CAD build for the part. Positions are in the model's coordinates, mm. A direction names the side the tool comes from. Coordinates: 2 decimals unless noted, no trailing zeros. Loops run counter-clockwise (first coordinate to the right, second up) from the corner with the lowest first, then second, coordinate; pieces in that order, holes last.
1) Which spindle directions (+Z, -Z, +X, -X, +Y, -Y) get a long thin tool onto all of the face, cutting with end or side? Do faces 1 (the flat face through (-14, 49.431, 5)), 2 (the flat face through (-1, -10, 10)), 3 (the flat face through (39, 49.431, 5)), 4 (the flat face through (-38, 49.431, 5)). Say none if no direction does.
2) Saw through at C-C, the plane x = -42. Write the cut outline in (y, z), and give its area (3 significant figures).
3) Two-plate mould, pull along Y, no slides. Class faces 5 (the flat face through (0, 8, 12)), 6 (the cylindrical face through (8.41, 44.34, 10.99)), 7 (the flat face through (-1, -49.431, 5)): +Y half, -Y half, draft (parallel to the pull), parting line (faces both ways), or undercut.
4) Saw through at A-A, the plane z = 3.25. Write the cut outline in (x, y), and give its area (3 significant figures).
5) Wall check: line 1 along X through (y, z) = (3, 10.5); line 2 along X through (y, z) = (4.5, 10.25); line 3 along Y through (x, z) = (13, 6.75). Give the ranges that are in metal, low to high.
6) Saw through at B-B, the plane y = 2. Write the cut outline in (x, z).
7) Saw through at D-D, the plane y = -42. Write the cut outline in (x, z).
8) Pin check, flat tips, straight feed: pin 1 Ø4 at (y, z) = (61.5, 8.5) entering from -X; pin 2 Ø6.5 at (x, z) = (14.5, 5) entering from +Y; pin 3 Ø4.5 at (x, z) = (-13, 6.5) entering from +Y. Stop position of each tip, or through.
```python
from build123d import *

# Parameters (mm, degrees)
F0_W     = 103.961334
F0_H     = 98.86241
F1_DEPTH = 10
F3_DEPTH = 2
F5_DEPTH = 2
F7_DEPTH = 12


with BuildPart() as f1:
    # F0 (on Top) → F1 (new body)
    with BuildSketch(Plane.XY):
        Rectangle(F0_W, F0_H)
    extrude(amount=F1_DEPTH)

    # F2 (on face) → F3 (join)
    with BuildSketch(Plane.XY.offset(10)):
        with BuildLine():
            ThreePointArc((-16.892111, 15.737094), (-21.169771, -9.210881), (0, -23.086783))
            ThreePointArc((0, -23.086783), (21.247464, -9.030216), (16.621562, 16.022585))
            Line((16.621562, 16.022585), (14.340605, 13.488688))
            ThreePointArc((14.340605, 13.488688), (18.071472, -7.811502), (0, -19.6875))
            ThreePointArc((0, -19.6875), (-18.227079, -7.441185), (-13.778395, 14.062485))
            Line((-13.778395, 14.062485), (-16.892111, 15.737094))
        make_face()
    extrude(amount=F3_DEPTH)

    # F4 (on face) → F5 (join)
    with BuildSketch(Plane.XY.offset(10)):
        with BuildLine():
            ThreePointArc((-3.965827, -3.950249), (-3.095911, -7.256054), (0, -8.70534))
            ThreePointArc((0, -8.70534), (3.095911, -7.256054), (3.965827, -3.950249))
            Line((3.965827, -3.950249), (3.965827, 20.820595))
            ThreePointArc((3.965827, 20.820595), (2.804263, 23.624858), (0, 24.786422))
            ThreePointArc((0, 24.786422), (-2.804263, 23.624858), (-3.965827, 20.820595))
            Line((-3.965827, 20.820595), (-3.965827, -3.950249))
        make_face()
    extrude(amount=F5_DEPTH)

    # F6 (on Top) → F7 (join)
    with BuildSketch(Plane.XY):
        with BuildLine():
            Line((10.162761, 64.030863), (0, 64.030863))
            Line((0, 64.030863), (-10.268303, 64.030863))
            Line((-10.268303, 64.030863), (-10.268303, 60.425382))
            Line((-10.268303, 60.425382), (-30.499062, 60.425382))
            Line((-30.499062, 60.425382), (-18.681094, 38.792491))
            ThreePointArc((-18.681094, 38.792491), (-15.118518, 37.676481), (-13.873785, 41.196149))
            Line((-13.873785, 41.196149), (-20.884443, 54.215942))
            Line((-20.884443, 54.215942), (-9.066476, 54.215942))
            Line((-9.066476, 54.215942), (-4.659776, 54.215942))
            Line((-4.659776, 54.215942), (6.356973, 54.215942))
            Line((6.356973, 54.215942), (10.56337, 54.215942))
            Line((10.56337, 54.215942), (20.578595, 54.215942))
            Line((20.578595, 54.215942), (15.170373, 40.795539))
            ThreePointArc((15.170373, 40.795539), (16.738154, 36.83037), (20.778898, 38.191579))
            Line((20.778898, 38.191579), (30.193213, 60.225077))
            Line((30.193213, 60.225077), (10.162761, 60.225077))
            Line((10.162761, 60.225077), (10.162761, 64.030863))
        make_face()
        with BuildLine():
            Line((10.56337, 46.804674), (10.56337, 54.215942))
            Line((10.56337, 54.215942), (6.356973, 54.215942))
            Line((6.356973, 54.215942), (6.356973, 46.804674))
            ThreePointArc((6.356973, 46.804674), (8.460172, 44.341305), (10.56337, 46.804674))
        make_face()
        with BuildLine():
            Line((-4.659776, 54.215942), (-9.066476, 54.215942))
            Line((-9.066476, 54.215942), (-9.066476, 46.604369))
            ThreePointArc((-9.066476, 46.604369), (-6.680204, 44.792543), (-4.659776, 47.004979))
            Line((-4.659776, 47.004979), (-4.659776, 54.215942))
        make_face()
    extrude(amount=F7_DEPTH)


solid = f1.part
```
Data:
1. face 1: +Z, -Z
1. face 2: +Z
1. face 3: +Z, -Z, +X
1. face 4: +Z, -Z, -X
2. outline: (-49.43, 0) - (49.43, 0) - (49.43, 10) - (-49.43, 10) - close
2. area: 989 mm2
3. face 5: draft
3. face 6: undercut
3. face 7: -Y half
4. outline: (-51.98, -49.43) - (51.98, -49.43) - (51.98, 49.43) - (25.58, 49.43) - (30.19, 60.23) - (10.16, 60.23) - (10.16, 64.03) - (-10.27, 64.03) - (-10.27, 60.43) - (-30.5, 60.43) - (-24.49, 49.43) - (-51.98, 49.43) - close; hole (-20.88, 54.22) - (-18.31, 49.43) - (-9.07, 49.43) - (-9.07, 54.22) - close; hole (-4.66, 49.43) - (6.36, 49.43) - (6.36, 54.22) - (-4.66, 54.22) - close; hole (10.56, 49.43) - (18.65, 49.43) - (20.58, 54.22) - (10.56, 54.22) - close
4. area: 10,800 mm2
5. line 1: x = -22.89 to -19.46, -3.97 to 3.97, 19.46 to 22.89
5. line 2: x = -22.64 to -19.17, -3.97 to 3.97, 19.17 to 22.64
5. line 3: y = -49.43 to 49.43, 54.22 to 60.23
6. outline: (-51.98, 0) - (51.98, 0) - (51.98, 10) - (23, 10) - (23, 12) - (19.59, 12) - (19.59, 10) - (3.97, 10) - (3.97, 12) - (-3.97, 12) - (-3.97, 10) - (-19.59, 10) - (-19.59, 12) - (-23, 12) - (-23, 10) - (-51.98, 10) - close
7. outline: (-51.98, 0) - (51.98, 0) - (51.98, 10) - (-51.98, 10) - close
8. pin 1: stops at x = -30.5
8. pin 2: stops at y = 60.23
8. pin 3: stops at y = 60.43
